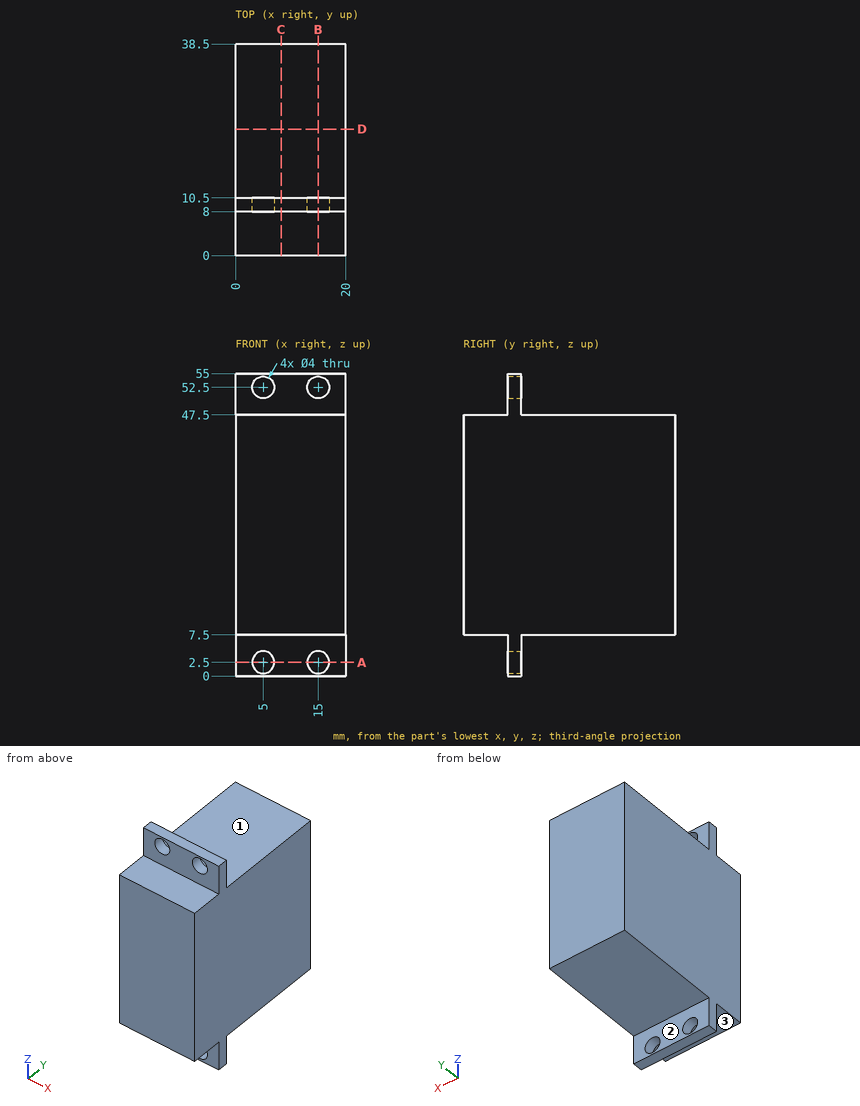
Geometry check sheet. Reference: drawing and pictorial views, mm from the part's lowest x, y, z. A direction names the side the tool comes from. Coordinates: 2 decimals unless noted, no trailing zeros. Write each loop counter-clockwise with the first axis right and the second up, starting at its lowest first coordinate (ties: lowest second). Pieces come first, ordered by that corner, then holes. Notation, with made-up numbers: (40.25, -4) - (81.25, -4) arc R22 cw to (81.25, 29) - close; hole circle Ø10 at (35.25, 65.5). An arc over 180 degrees is marked (long way). One line per question, with ' | ' between items. Start each with the question number.
1. Section check C-C (x = 8.25). Enter the section's corners in (y, z).
2. Material ranges on line 1 along Z through (x, y) = (15, 8.9); line 2 along X through (y, z) = (8.6, 52.5); line 3 along X through (y, z) = (10, 2), recorded low to high.
3. Section check D-D (y = 23). Enter the section's corners in (x, z).
4. Access from +Z, -Z, +X, -X, +Y, -Y to the whole of each face (thin tool, end or side, straight path). Record for the marked faces 1, 2 and 3.
5. Section check B-B (x = 15). Enter the section's corners in (y, z).
6. Section check A-A (z = 2.5). Enter the section's corners in (x, y).
7. Gauge pin test, flat ends, axial feed: P1, Ø4, axis at x = 7, z = 51.5, coming from the -Y side; P2, Ø1.5, axis at x = 9.5, y = 31, coming from the -Z side; P3, Ø4, axis at x = 6.5, z = 5, coming from the +Y side. Record the tip position at first contact, or that the pin passes through.
Computed values:
1) outline: (0, 7.5) - (8, 7.5) - (8, 0) - (10.5, 0) - (10.5, 7.5) - (38.5, 7.5) - (38.5, 47.5) - (10.5, 47.5) - (10.5, 55) - (8, 55) - (8, 47.5) - (0, 47.5) - close
2) line 1: 0 to 0.5, 4.5 to 50.5, 54.5 to 55 | line 2: 0 to 3, 7 to 13, 17 to 20 | line 3: 0 to 3.06, 6.94 to 13.06, 16.94 to 20
3) outline: (0, 7.5) - (20, 7.5) - (20, 47.5) - (0, 47.5) - close
4) face 1: +Z, +X, -X, +Y | face 2: -Z, +X, -X, +Y | face 3: -Z, +X, -X, -Y
5) outline: (0, 7.5) - (8, 7.5) - (8, 4.5) - (10.5, 4.5) - (10.5, 7.5) - (38.5, 7.5) - (38.5, 47.5) - (10.5, 47.5) - (10.5, 50.5) - (8, 50.5) - (8, 47.5) - (0, 47.5) - close; (8, 0) - (10.5, 0) - (10.5, 0.5) - (8, 0.5) - close; (8, 54.5) - (10.5, 54.5) - (10.5, 55) - (8, 55) - close
6) outline: (0, 8) - (3, 8) - (3, 10.5) - (0, 10.5) - close; (7, 8) - (13, 8) - (13, 10.5) - (7, 10.5) - close; (17, 8) - (20, 8) - (20, 10.5) - (17, 10.5) - close
7) P1: y = 8 | P2: z = 7.5 | P3: y = 10.5
